Source: CAD feature listing. Evaluate the final solid. Frame: model axes, mm. Coordinates: 2 decimals unless noted, no trailing zeros. Write each loop counter-clockwise with the first axis right and the second up, starting at its lowest first coordinate (ties: lowest second). Pieces come first, ordered by that corner, then holes. Notation, with made-up numbers: (58.25, 74.25) - (90.25, 74.25) arc R24 cw to (90.25, 112.25) - close; hole circle Ø9 at (25, 10.5). An arc over 180 degrees is marked (long way). One line per item, written item: value.
from build123d import *

# Parameters (mm, degrees)
SKETCH_2_W                        = 1000
SKETCH_2_H                        = 1160
EXTRUDE_1_DEPTH                   = 16
CUT_EXTRUDE_1_DEPTH               = 766.934723067
SKETCH_6_R                        = 13
CUT_EXTRUDE_2_DEPTH               = 766.934723067
PATTERN_LINEAR_1_COUNT            = 4
PATTERN_LINEAR_1_PITCH            = 80
PATTERN_LINEAR_1_COUNT_DIR2       = 3
PATTERN_LINEAR_1_PITCH_DIR2       = 80
PATTERN_LINEAR_2_COUNT            = 2
PATTERN_LINEAR_2_PITCH            = 360
PATTERN_LINEAR_2_COPY_1_SKETCH_R  = 13
PATTERN_LINEAR_2_COPY_1_DEPTH     = 766.934723067
PATTERN_LINEAR_2_COPY_2_SKETCH_R  = 13
PATTERN_LINEAR_2_COPY_2_DEPTH     = 766.934723067
PATTERN_LINEAR_2_COPY_3_SKETCH_R  = 13
PATTERN_LINEAR_2_COPY_3_DEPTH     = 766.934723067
PATTERN_LINEAR_2_COPY_4_SKETCH_R  = 13
PATTERN_LINEAR_2_COPY_4_DEPTH     = 766.934723067
PATTERN_LINEAR_2_COPY_5_SKETCH_R  = 13
PATTERN_LINEAR_2_COPY_5_DEPTH     = 766.934723067
PATTERN_LINEAR_2_COPY_6_SKETCH_R  = 13
PATTERN_LINEAR_2_COPY_6_DEPTH     = 766.934723067
PATTERN_LINEAR_2_COPY_7_SKETCH_R  = 13
PATTERN_LINEAR_2_COPY_7_DEPTH     = 766.934723067
PATTERN_LINEAR_2_COPY_8_SKETCH_R  = 13
PATTERN_LINEAR_2_COPY_8_DEPTH     = 766.934723067
PATTERN_LINEAR_2_COPY_9_SKETCH_R  = 13
PATTERN_LINEAR_2_COPY_9_DEPTH     = 766.934723067
PATTERN_LINEAR_2_COPY_10_SKETCH_R = 13
PATTERN_LINEAR_2_COPY_10_DEPTH    = 766.934723067
PATTERN_LINEAR_2_COPY_11_SKETCH_R = 13
PATTERN_LINEAR_2_COPY_11_DEPTH    = 766.934723067
SKETCH_7_R                        = 13
CUT_EXTRUDE_3_DEPTH               = 766.934723067
PATTERN_LINEAR_3_COUNT            = 3
PATTERN_LINEAR_3_PITCH            = 56
PATTERN_LINEAR_3_COUNT_DIR2       = 3
PATTERN_LINEAR_3_PITCH_DIR2       = 80
PATTERN_LINEAR_4_COUNT            = 2
PATTERN_LINEAR_4_PITCH            = 800
PATTERN_LINEAR_4_COPY_1_SKETCH_R  = 13
PATTERN_LINEAR_4_COPY_1_DEPTH     = 766.934723067
PATTERN_LINEAR_4_COPY_2_SKETCH_R  = 13
PATTERN_LINEAR_4_COPY_2_DEPTH     = 766.934723067
PATTERN_LINEAR_4_COPY_3_SKETCH_R  = 13
PATTERN_LINEAR_4_COPY_3_DEPTH     = 766.934723067
PATTERN_LINEAR_4_COPY_4_SKETCH_R  = 13
PATTERN_LINEAR_4_COPY_4_DEPTH     = 766.934723067
PATTERN_LINEAR_4_COPY_5_SKETCH_R  = 13
PATTERN_LINEAR_4_COPY_5_DEPTH     = 766.934723067
PATTERN_LINEAR_4_COPY_6_SKETCH_R  = 13
PATTERN_LINEAR_4_COPY_6_DEPTH     = 766.934723067
PATTERN_LINEAR_4_COPY_7_SKETCH_R  = 13
PATTERN_LINEAR_4_COPY_7_DEPTH     = 766.934723067
PATTERN_LINEAR_4_COPY_8_SKETCH_R  = 13
PATTERN_LINEAR_4_COPY_8_DEPTH     = 766.934723067
SKETCH_8_R                        = 13
CUT_EXTRUDE_4_DEPTH               = 766.934723067
MIRROR_2_COPY_1_SKETCH_R          = 13
MIRROR_2_COPY_1_DEPTH             = 766.934723067


with BuildPart() as part:
    # 草图2 → 凸台-拉伸1 (new body)
    with BuildSketch(Plane.XY):
        Rectangle(SKETCH_2_W, SKETCH_2_H)
    extrude(amount=EXTRUDE_1_DEPTH)

    # 草图4 → 切除-拉伸1 (cut, through all)
    with BuildSketch(Plane(origin=(0, 0, 0), x_dir=(-1, 0, 0), z_dir=(0, 0, -1))):
        Polygon((-500, 360), (-430, 180), (-430, -180), (-500, -360), align=None)
        Polygon((430, 180), (430, -180), (500, -360), (500, 360), align=None)
    extrude(amount=-CUT_EXTRUDE_1_DEPTH, mode=Mode.SUBTRACT)

    # 草图6 → 切除-拉伸2 (cut, through all)
    with BuildSketch(Plane.XY.offset(16)):
        with Locations((-60, 80)):
            Circle(SKETCH_6_R)
    cut_extrude_2 = extrude(amount=-CUT_EXTRUDE_2_DEPTH, mode=Mode.SUBTRACT)

    # 阵列(线性)1: Cut-Extrude 2 4 × 3
    with Locations(*[(-i * PATTERN_LINEAR_1_PITCH, -j * PATTERN_LINEAR_1_PITCH_DIR2, 0) for i in range(PATTERN_LINEAR_1_COUNT) for j in range(PATTERN_LINEAR_1_COUNT_DIR2) if (i, j) != (0, 0)]):
        add(cut_extrude_2, mode=Mode.SUBTRACT)

    # 阵列(线性)2: 切除-拉伸2 ×2
    with Locations(*[(i * PATTERN_LINEAR_2_PITCH, 0, 0) for i in range(1, PATTERN_LINEAR_2_COUNT)]):
        add(cut_extrude_2, mode=Mode.SUBTRACT)

    # 阵列(线性)2 copy 1 sketch → 阵列(线性)2 copy 1 (cut, through all)
    with BuildSketch(Plane(origin=(360, -80, 16), x_dir=(1, 0, 0), z_dir=(0, 0, 1))):
        with Locations((-60, 80)):
            Circle(PATTERN_LINEAR_2_COPY_1_SKETCH_R)
    extrude(amount=-PATTERN_LINEAR_2_COPY_1_DEPTH, mode=Mode.SUBTRACT)

    # 阵列(线性)2 copy 2 sketch → 阵列(线性)2 copy 2 (cut, through all)
    with BuildSketch(Plane(origin=(360, -160, 16), x_dir=(1, 0, 0), z_dir=(0, 0, 1))):
        with Locations((-60, 80)):
            Circle(PATTERN_LINEAR_2_COPY_2_SKETCH_R)
    extrude(amount=-PATTERN_LINEAR_2_COPY_2_DEPTH, mode=Mode.SUBTRACT)

    # 阵列(线性)2 copy 3 sketch → 阵列(线性)2 copy 3 (cut, through all)
    with BuildSketch(Plane(origin=(280, 0, 16), x_dir=(1, 0, 0), z_dir=(0, 0, 1))):
        with Locations((-60, 80)):
            Circle(PATTERN_LINEAR_2_COPY_3_SKETCH_R)
    extrude(amount=-PATTERN_LINEAR_2_COPY_3_DEPTH, mode=Mode.SUBTRACT)

    # 阵列(线性)2 copy 4 sketch → 阵列(线性)2 copy 4 (cut, through all)
    with BuildSketch(Plane(origin=(280, -80, 16), x_dir=(1, 0, 0), z_dir=(0, 0, 1))):
        with Locations((-60, 80)):
            Circle(PATTERN_LINEAR_2_COPY_4_SKETCH_R)
    extrude(amount=-PATTERN_LINEAR_2_COPY_4_DEPTH, mode=Mode.SUBTRACT)

    # 阵列(线性)2 copy 5 sketch → 阵列(线性)2 copy 5 (cut, through all)
    with BuildSketch(Plane(origin=(280, -160, 16), x_dir=(1, 0, 0), z_dir=(0, 0, 1))):
        with Locations((-60, 80)):
            Circle(PATTERN_LINEAR_2_COPY_5_SKETCH_R)
    extrude(amount=-PATTERN_LINEAR_2_COPY_5_DEPTH, mode=Mode.SUBTRACT)

    # 阵列(线性)2 copy 6 sketch → 阵列(线性)2 copy 6 (cut, through all)
    with BuildSketch(Plane(origin=(200, 0, 16), x_dir=(1, 0, 0), z_dir=(0, 0, 1))):
        with Locations((-60, 80)):
            Circle(PATTERN_LINEAR_2_COPY_6_SKETCH_R)
    extrude(amount=-PATTERN_LINEAR_2_COPY_6_DEPTH, mode=Mode.SUBTRACT)

    # 阵列(线性)2 copy 7 sketch → 阵列(线性)2 copy 7 (cut, through all)
    with BuildSketch(Plane(origin=(200, -80, 16), x_dir=(1, 0, 0), z_dir=(0, 0, 1))):
        with Locations((-60, 80)):
            Circle(PATTERN_LINEAR_2_COPY_7_SKETCH_R)
    extrude(amount=-PATTERN_LINEAR_2_COPY_7_DEPTH, mode=Mode.SUBTRACT)

    # 阵列(线性)2 copy 8 sketch → 阵列(线性)2 copy 8 (cut, through all)
    with BuildSketch(Plane(origin=(200, -160, 16), x_dir=(1, 0, 0), z_dir=(0, 0, 1))):
        with Locations((-60, 80)):
            Circle(PATTERN_LINEAR_2_COPY_8_SKETCH_R)
    extrude(amount=-PATTERN_LINEAR_2_COPY_8_DEPTH, mode=Mode.SUBTRACT)

    # 阵列(线性)2 copy 9 sketch → 阵列(线性)2 copy 9 (cut, through all)
    with BuildSketch(Plane(origin=(120, 0, 16), x_dir=(1, 0, 0), z_dir=(0, 0, 1))):
        with Locations((-60, 80)):
            Circle(PATTERN_LINEAR_2_COPY_9_SKETCH_R)
    extrude(amount=-PATTERN_LINEAR_2_COPY_9_DEPTH, mode=Mode.SUBTRACT)

    # 阵列(线性)2 copy 10 sketch → 阵列(线性)2 copy 10 (cut, through all)
    with BuildSketch(Plane(origin=(120, -80, 16), x_dir=(1, 0, 0), z_dir=(0, 0, 1))):
        with Locations((-60, 80)):
            Circle(PATTERN_LINEAR_2_COPY_10_SKETCH_R)
    extrude(amount=-PATTERN_LINEAR_2_COPY_10_DEPTH, mode=Mode.SUBTRACT)

    # 阵列(线性)2 copy 11 sketch → 阵列(线性)2 copy 11 (cut, through all)
    with BuildSketch(Plane(origin=(120, -160, 16), x_dir=(1, 0, 0), z_dir=(0, 0, 1))):
        with Locations((-60, 80)):
            Circle(PATTERN_LINEAR_2_COPY_11_SKETCH_R)
    extrude(amount=-PATTERN_LINEAR_2_COPY_11_DEPTH, mode=Mode.SUBTRACT)

    # 草图7 → 切除-拉伸3 (cut, through all)
    with BuildSketch(Plane.XY.offset(16)):
        with Locations((-56, 480)):
            Circle(SKETCH_7_R)
    cut_extrude_3 = extrude(amount=-CUT_EXTRUDE_3_DEPTH, mode=Mode.SUBTRACT)

    # 阵列(线性)3: Cut-Extrude 3 3 × 3
    with Locations(*[(i * PATTERN_LINEAR_3_PITCH, -j * PATTERN_LINEAR_3_PITCH_DIR2, 0) for i in range(PATTERN_LINEAR_3_COUNT) for j in range(PATTERN_LINEAR_3_COUNT_DIR2) if (i, j) != (0, 0)]):
        add(cut_extrude_3, mode=Mode.SUBTRACT)

    # 阵列(线性)4: 切除-拉伸3 ×2
    with Locations(*[(0, -i * PATTERN_LINEAR_4_PITCH, 0) for i in range(1, PATTERN_LINEAR_4_COUNT)]):
        add(cut_extrude_3, mode=Mode.SUBTRACT)

    # 阵列(线性)4 copy 1 sketch → 阵列(线性)4 copy 1 (cut, through all)
    with BuildSketch(Plane(origin=(0, -880, 16), x_dir=(1, 0, 0), z_dir=(0, 0, 1))):
        with Locations((-56, 480)):
            Circle(PATTERN_LINEAR_4_COPY_1_SKETCH_R)
    extrude(amount=-PATTERN_LINEAR_4_COPY_1_DEPTH, mode=Mode.SUBTRACT)

    # 阵列(线性)4 copy 2 sketch → 阵列(线性)4 copy 2 (cut, through all)
    with BuildSketch(Plane(origin=(0, -960, 16), x_dir=(1, 0, 0), z_dir=(0, 0, 1))):
        with Locations((-56, 480)):
            Circle(PATTERN_LINEAR_4_COPY_2_SKETCH_R)
    extrude(amount=-PATTERN_LINEAR_4_COPY_2_DEPTH, mode=Mode.SUBTRACT)

    # 阵列(线性)4 copy 3 sketch → 阵列(线性)4 copy 3 (cut, through all)
    with BuildSketch(Plane(origin=(56, -800, 16), x_dir=(1, 0, 0), z_dir=(0, 0, 1))):
        with Locations((-56, 480)):
            Circle(PATTERN_LINEAR_4_COPY_3_SKETCH_R)
    extrude(amount=-PATTERN_LINEAR_4_COPY_3_DEPTH, mode=Mode.SUBTRACT)

    # 阵列(线性)4 copy 4 sketch → 阵列(线性)4 copy 4 (cut, through all)
    with BuildSketch(Plane(origin=(56, -880, 16), x_dir=(1, 0, 0), z_dir=(0, 0, 1))):
        with Locations((-56, 480)):
            Circle(PATTERN_LINEAR_4_COPY_4_SKETCH_R)
    extrude(amount=-PATTERN_LINEAR_4_COPY_4_DEPTH, mode=Mode.SUBTRACT)

    # 阵列(线性)4 copy 5 sketch → 阵列(线性)4 copy 5 (cut, through all)
    with BuildSketch(Plane(origin=(56, -960, 16), x_dir=(1, 0, 0), z_dir=(0, 0, 1))):
        with Locations((-56, 480)):
            Circle(PATTERN_LINEAR_4_COPY_5_SKETCH_R)
    extrude(amount=-PATTERN_LINEAR_4_COPY_5_DEPTH, mode=Mode.SUBTRACT)

    # 阵列(线性)4 copy 6 sketch → 阵列(线性)4 copy 6 (cut, through all)
    with BuildSketch(Plane(origin=(112, -800, 16), x_dir=(1, 0, 0), z_dir=(0, 0, 1))):
        with Locations((-56, 480)):
            Circle(PATTERN_LINEAR_4_COPY_6_SKETCH_R)
    extrude(amount=-PATTERN_LINEAR_4_COPY_6_DEPTH, mode=Mode.SUBTRACT)

    # 阵列(线性)4 copy 7 sketch → 阵列(线性)4 copy 7 (cut, through all)
    with BuildSketch(Plane(origin=(112, -880, 16), x_dir=(1, 0, 0), z_dir=(0, 0, 1))):
        with Locations((-56, 480)):
            Circle(PATTERN_LINEAR_4_COPY_7_SKETCH_R)
    extrude(amount=-PATTERN_LINEAR_4_COPY_7_DEPTH, mode=Mode.SUBTRACT)

    # 阵列(线性)4 copy 8 sketch → 阵列(线性)4 copy 8 (cut, through all)
    with BuildSketch(Plane(origin=(112, -960, 16), x_dir=(1, 0, 0), z_dir=(0, 0, 1))):
        with Locations((-56, 480)):
            Circle(PATTERN_LINEAR_4_COPY_8_SKETCH_R)
    extrude(amount=-PATTERN_LINEAR_4_COPY_8_DEPTH, mode=Mode.SUBTRACT)

    # 草图8 → 切除-拉伸4 (cut, through all)
    with BuildSketch(Plane.XY.offset(16)):
        with Locations((175.539308363, 347.486620202)):
            Circle(SKETCH_8_R)
        with Locations((300.478317874, 247.535412593)):
            Circle(SKETCH_8_R)
        with Locations((225.514912167, 409.956124958)):
            Circle(SKETCH_8_R)
        with Locations((275.490515972, 472.425629713)):
            Circle(SKETCH_8_R)
        with Locations((325.466119776, 534.895134468)):
            Circle(SKETCH_8_R)
        with Locations((387.935624531, 484.919530664)):
            Circle(SKETCH_8_R)
        with Locations((337.960020727, 422.450025909)):
            Circle(SKETCH_8_R)
        with Locations((287.984416923, 359.980521153)):
            Circle(SKETCH_8_R)
        with Locations((450.405129287, 434.94392686)):
            Circle(SKETCH_8_R)
        with Locations((400.429525482, 372.474422104)):
            Circle(SKETCH_8_R)
        with Locations((350.453921678, 310.004917349)):
            Circle(SKETCH_8_R)
        with Locations((238.008813118, 297.511016398)):
            Circle(SKETCH_8_R)
    cut_extrude_4 = extrude(amount=-CUT_EXTRUDE_4_DEPTH, mode=Mode.SUBTRACT)

    # 镜向1: 切除-拉伸4 across plane
    add(cut_extrude_4.mirror(Plane(origin=(0, 0, 0), x_dir=(0, 0, 1), z_dir=(1, 0, 0))), mode=Mode.SUBTRACT)

    # 镜向2: 切除-拉伸4 across plane
    add(cut_extrude_4.mirror(Plane.ZX), mode=Mode.SUBTRACT)

    # 镜向2 copy 1 sketch → 镜向2 copy 1 (cut, through all)
    with BuildSketch(Plane(origin=(0, 0, 16), x_dir=(-1, 0, 0), z_dir=(0, 0, 1))):
        with Locations((175.539308363, 347.486620202)):
            Circle(MIRROR_2_COPY_1_SKETCH_R)
        with Locations((300.478317874, 247.535412593)):
            Circle(MIRROR_2_COPY_1_SKETCH_R)
        with Locations((225.514912167, 409.956124958)):
            Circle(MIRROR_2_COPY_1_SKETCH_R)
        with Locations((275.490515972, 472.425629713)):
            Circle(MIRROR_2_COPY_1_SKETCH_R)
        with Locations((325.466119776, 534.895134468)):
            Circle(MIRROR_2_COPY_1_SKETCH_R)
        with Locations((387.935624531, 484.919530664)):
            Circle(MIRROR_2_COPY_1_SKETCH_R)
        with Locations((337.960020727, 422.450025909)):
            Circle(MIRROR_2_COPY_1_SKETCH_R)
        with Locations((287.984416923, 359.980521153)):
            Circle(MIRROR_2_COPY_1_SKETCH_R)
        with Locations((450.405129287, 434.94392686)):
            Circle(MIRROR_2_COPY_1_SKETCH_R)
        with Locations((400.429525482, 372.474422104)):
            Circle(MIRROR_2_COPY_1_SKETCH_R)
        with Locations((350.453921678, 310.004917349)):
            Circle(MIRROR_2_COPY_1_SKETCH_R)
        with Locations((238.008813118, 297.511016398)):
            Circle(MIRROR_2_COPY_1_SKETCH_R)
    extrude(amount=-MIRROR_2_COPY_1_DEPTH, mode=Mode.SUBTRACT)


solid = part.part
1) Material intervals for line 1 (X direction, y = -438.5, z = 10); line 2 (Y direction, x = -210, z = 9.5); line 3 (Y direction, x = 359, z = 13), sorted ascending.
Values found:
line 1: -500 to -462.91, -437.9 to 437.9, 462.91 to 500
line 2: -580 to -88.31, -71.69 to -8.31, 8.31 to 71.69, 88.31 to 580
line 3: -580 to -319.8, -300.21 to 300.21, 319.8 to 580
2) Contact query for flat-ended pins moving along their axis: P1, Ø15.5, axis at x = 0, y = 320, coming from the -Z side; P2, Ø2, axis at x = 208, y = 28, coming from the -Z side. Output: stop coordinate, or through.
Values found:
P1: through
P2: z = 0
3) Section query A-A on x = 140. Output: boundary loops of the cut face in (y, z), then the cut area to 3 significant figures.
Values found:
outline: (-580, 0) - (-93, 0) - (-93, 16) - (-580, 16) - close; (-67, 0) - (-13, 0) - (-13, 16) - (-67, 16) - close; (13, 0) - (67, 0) - (67, 16) - (13, 16) - close; (93, 0) - (580, 0) - (580, 16) - (93, 16) - close
area: 17,300 mm2
4) Section query B-B on x = 0. Output: boundary loops of the cut face in (y, z), then the cut area to 3 significant figures.
Values found:
outline: (-580, 0) - (-493, 0) - (-493, 16) - (-580, 16) - close; (-467, 0) - (-413, 0) - (-413, 16) - (-467, 16) - close; (-387, 0) - (-333, 0) - (-333, 16) - (-387, 16) - close; (-307, 0) - (307, 0) - (307, 16) - (-307, 16) - close; (333, 0) - (387, 0) - (387, 16) - (333, 16) - close; (413, 0) - (467, 0) - (467, 16) - (413, 16) - close; (493, 0) - (580, 0) - (580, 16) - (493, 16) - close
area: 16,100 mm2
5) Section query C-C on y = 80. State how many separate pieces and enclosed holes the cut face has, then the cut area to 3 significant figures.
Values found:
separate pieces: 9
enclosed holes: 0
area: 10,400 mm2
